Input: part model. Units: mm. Frame: model coordinates. Face numbers are marked on the shaded views. A direction names the side the tool comes from. Round coordinates to 2 decimals unless told otherwise and drop trailing zeros. Order: outer loops, then holes, each group sorted by start corner. A loop starts at its lowest first (then second) coordinate and runs counter-clockwise, first axis right, second up. Notation, with made-up numbers: (-30.75, 21) - (-1.75, 21) arc R4 cw to (-1.75, 25) - close; hole circle Ø10 at (80, -19.5). An arc over 180 degrees is marked (long way). One line per item, written item: value. Start each with the question number.
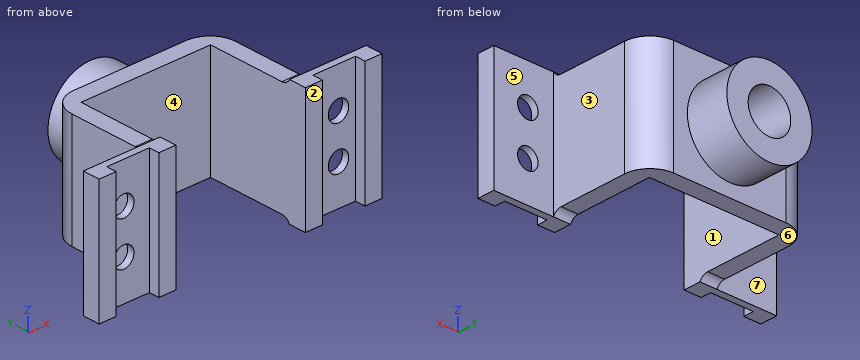
from build123d import *

# Parameters (mm, degrees)
SKETCH1_W           = 96
SKETCH1_H           = 70
BOSS_EXTRUDE1_DEPTH = 32.5
BOSS_EXTRUDE2_DEPTH = 35.5
SKETCH3_W           = 76
SKETCH3_H           = 60
CUT_EXTRUDE1_DEPTH  = 129.113231167
FILLET1_R           = 15
FILLET2_R           = 5.5
SKETCH4_R           = 25
SKETCH4_R_2         = 12.5
BOSS_EXTRUDE3_DEPTH = 25
HOLE1_D             = 12


with BuildPart() as part:
    # Sketch1 → Boss-Extrude1 (new, symmetric)
    with BuildSketch(Plane.XY):
        with Locations((0, 35)):
            Rectangle(SKETCH1_W, SKETCH1_H)
    extrude(amount=BOSS_EXTRUDE1_DEPTH, both=True)

    # Sketch2 → Boss-Extrude2 (add, symmetric)
    with BuildSketch(Plane.XY):
        Polygon((38, 0), (38, 10), (83, 10), (83, 0), (73, 0), (73, 6), (48, 6), (48, 0), align=None)
    boss_extrude2 = extrude(amount=BOSS_EXTRUDE2_DEPTH, both=True)

    # Mirror1: Boss-Extrude2 across plane
    add(boss_extrude2.mirror(Plane(origin=(0, 0, 0), x_dir=(0, 0, 1), z_dir=(1, 0, 0))))

    # Sketch3 → Cut-Extrude1 (cut, through all)
    with BuildSketch(Plane.XY.offset(32.5)):
        with Locations((0, 30)):
            Rectangle(SKETCH3_W, SKETCH3_H)
    extrude(amount=-CUT_EXTRUDE1_DEPTH, mode=Mode.SUBTRACT)

    # Fillet1
    fillet1_edges = [part.edges().sort_by_distance(p)[0] for p in [
        (-48, 70, 0),
        (48, 70, 0),
    ]]
    fillet(fillet1_edges, radius=FILLET1_R)

    # Fillet2
    # the kernel refuses this fillet: 5.5 mm, written as the material it adds along each edge
    with BuildSketch(Plane(origin=(-48, 10, -32.5), x_dir=(0, 1, 0), z_dir=(1, 0, 0)), Plane(origin=(48, 10, 32.5), x_dir=(0, 1, 0), z_dir=(-1, 0, 0))) as fillet2_piece_1:
        with BuildLine():
            CenterArc((4.898979486, -5.5), FILLET2_R, 90, 62.964308211)
            Line((0, -3), (-0.09797959, -2.95))
            ThreePointArc((-0.09797959, -2.95), (-0.11, -1.5), (-0.11, 0))
            Line((-0.11, 0), (0, 0.11))
            Line((0, 0.11), (4.898979486, 0.11))
            Line((4.898979486, 0.11), (4.898979486, 0))
        make_face()
    extrude(amount=10)
    with BuildSketch(Plane(origin=(48, 10, -32.5), x_dir=(0, 1, 0), z_dir=(-1, 0, 0)), Plane(origin=(-48, 10, 32.5), x_dir=(0, 1, 0), z_dir=(1, 0, 0))) as fillet2_piece_2:
        with BuildLine():
            CenterArc((4.898979486, 5.5), FILLET2_R, 207.035691789, 62.964308211)
            Line((0, 3), (-0.09797959, 2.95))
            ThreePointArc((-0.09797959, 2.95), (-0.11, 1.5), (-0.11, 0))
            Line((-0.11, 0), (0, -0.11))
            Line((0, -0.11), (4.898979486, -0.11))
            Line((4.898979486, -0.11), (4.898979486, 0))
        make_face()
    extrude(amount=10)

    # Sketch4 → Boss-Extrude3 (add)
    with BuildSketch(Plane(origin=(0, 70, 0), x_dir=(1, 0, 0), z_dir=(0, 1, 0))):
        with Locations(Location((0, 0, 0), (0, 0, 270))):
            Circle(SKETCH4_R)
        with Locations(Location((0, 0, 0), (0, 0, 270))):
            Circle(SKETCH4_R_2, mode=Mode.SUBTRACT)
    extrude(amount=BOSS_EXTRUDE3_DEPTH)

    # Hole1 (through all)
    with Locations(Plane(origin=(0, 10, 0), x_dir=(1, 0, 0), z_dir=(0, 1, 0))):
        with Locations((63, 12.5), (63, -12.5)):
            hole1 = Hole(HOLE1_D / 2)

    # Mirror2: Hole1 across plane
    add(hole1.mirror(Plane(origin=(0, 0, 0), x_dir=(0, 0, 1), z_dir=(1, 0, 0))), mode=Mode.SUBTRACT)


solid = part.part
1. Section A-A (x = -63). Return the cut outline in (y, z), then the cut area to 3 significant figures.
2. Pin query (flat end, axial travel): pin 1 (3 mm diameter, centred on x = -24.5, z = -7, fed in from +Y); pin 2 (11 mm diameter, centred on x = -63, z = -12.5, fed in from +Y); pin 3 (18 mm diameter, centred on y = 22, z = -7, fed in from -X); pin 4 (1.5 mm diameter, centred on x = -22, z = 15.5, fed in from -Y). Return the tip coordinate at first contact, or that it passes through.
3. Section D-D (x = 64.5). Return the cut outline in (y, z).
4. Line query: line 1 (Z direction, x = 63, y = 8.85); line 2 (X direction, y = 9, z = -12); line 3 (X direction, y = 16.5, z = -16). Output: solid intervals per line, ascending. Write a range as from..to.
5. Section C-C (x = 0). Return the cut outline in (y, z), then the cut area to 4 significant figures.
6. Set-up query: the marked faces 4, 5, 6 and 7. Return all of +Z, -Z, +X, -X, +Y, -Y with unobstructed straight access to the full face (end or side cutting, diameter ignored); none if empty.
7. Pull-direction query (X, two-part tool) for the marked faces 1, 2 and 3; classes: released by +X, released by -X, zero draft, split by the parting line, or undercut.
Solved:
1. outline: (6, -35.5) - (10, -35.5) - (10, -18.5) - (6, -18.5) - close; (6, -6.5) - (10, -6.5) - (10, 6.5) - (6, 6.5) - close; (6, 18.5) - (10, 18.5) - (10, 35.5) - (6, 35.5) - close
1. area: 188 mm²
2. pin 1: stops at y = 95
2. pin 2: passes through
2. pin 3: stops at x = -48
2. pin 4: stops at y = 60
3. outline: (6, -35.5) - (10, -35.5) - (10, -18.31) - (6, -18.31) - close; (6, -6.69) - (10, -6.69) - (10, 6.69) - (6, 6.69) - close; (6, 18.31) - (10, 18.31) - (10, 35.5) - (6, 35.5) - close
4. line 1: z = -35.5..-18.5, -6.5..6.5, 18.5..35.5
4. line 2: x = -83..-68.98, -57.02..-38, 38..57.02, 68.98..83
4. line 3: x = -48..-38, 38..48
5. outline: (60, -32.5) - (70, -32.5) - (70, -25) - (95, -25) - (95, -12.5) - (70, -12.5) - (70, 12.5) - (95, 12.5) - (95, 25) - (70, 25) - (70, 32.5) - (60, 32.5) - close
5. area: 1,275 mm²
6. face 4: +Z, -Z, -Y
6. face 5: +Z, -Z, +X, +Y
6. face 6: -Z, +X, -X, +Y
6. face 7: +Z, -Z, -X, +Y
7. face 1: undercut
7. face 2: zero draft
7. face 3: released by +X
